from build123d import *

# Parameters (mm, degrees)
BOSS_EXTRUDE1_DEPTH        = 6.35
SKETCH2_R                  = 7
MOTOR_BEARING_HOLES_DEPTH  = 135.10382172
SKETCH3_R                  = 14.2875
CUT_EXTRUDE1_DEPTH         = 135.10382172
SKETCH4_R                  = 14.2875
CUT_EXTRUDE2_DEPTH         = 135.10382172
SKETCH5_R                  = 4.7625
CUT_EXTRUDE3_DEPTH         = 50.8
F_10_CLEARANCE_HOLE1_D     = 5.1054
F_10_CLEARANCE_HOLE2_D     = 5.1054
F_10_CLEARANCE_HOLE2_DEPTH = 50.8
F_10_CLEARANCE_HOLE2_TIP   = 1.533816902
FILLET1_R                  = 6.35
SKETCH10_R                 = 4.7625
CUT_EXTRUDE4_DEPTH         = 50.8


with BuildPart() as part:
    # Sketch1 → Boss-Extrude1 (new body)
    with BuildSketch(Plane(origin=(0, 0, 0), x_dir=(1, 0, 0), z_dir=(0, 1, 0))):
        Polygon((-69.85, -19.05), (69.85, -19.05), (69.85, 57.15), (6.35, 114.3), (-6.35, 114.3), (-69.85, 57.15), align=None)
    extrude(amount=BOSS_EXTRUDE1_DEPTH)

    # Sketch2 → Motor Bearing Holes (cut, through all)
    with BuildSketch(Plane(origin=(0, 6.35, 0), x_dir=(1, 0, 0), z_dir=(0, 1, 0))):
        with Locations(Location((-34.29, 25.4, 0), (0, 0, 270))):
            Circle(SKETCH2_R)
        with Locations(Location((34.29, 25.4, 0), (0, 0, 270))):
            Circle(SKETCH2_R)
    extrude(amount=-MOTOR_BEARING_HOLES_DEPTH, mode=Mode.SUBTRACT)

    # Sketch3 → Cut-Extrude1 (cut, through all)
    with BuildSketch(Plane(origin=(0, 6.35, 0), x_dir=(1, 0, 0), z_dir=(0, 1, 0))):
        with Locations(Location((0, 25.4, 0), (0, 0, 270))):
            Circle(SKETCH3_R)
    extrude(amount=-CUT_EXTRUDE1_DEPTH, mode=Mode.SUBTRACT)

    # Sketch4 → Cut-Extrude2 (cut, through all)
    with BuildSketch(Plane(origin=(0, 6.35, 0), x_dir=(1, 0, 0), z_dir=(0, 1, 0))):
        with Locations(Location((0, 63.5, 0), (0, 0, 270))):
            Circle(SKETCH4_R)
    extrude(amount=-CUT_EXTRUDE2_DEPTH, mode=Mode.SUBTRACT)

    # Sketch5 → Cut-Extrude3 (cut)
    with BuildSketch(Plane(origin=(0, 38.1, 19.05), x_dir=(-0.9584281674521108, 0, 0.2853339233851958), z_dir=(0, 1, 0))):
        with Locations(Location((21.697168114, -77.740965053, 0), (0, 0, 73.42119018))):
            Circle(SKETCH5_R)
        with Locations(Location((18.665649821, -27.031499499, 0), (0, 0, 73.42119018))):
            Circle(SKETCH5_R)
        with Locations(Location((-30.411025551, -12.420868461, 0), (0, 0, 73.42119018))):
            Circle(SKETCH5_R)
        with Locations(Location((-60.684163962, -53.21519516, 0), (0, 0, 73.42119018))):
            Circle(SKETCH5_R)
    extrude(amount=-CUT_EXTRUDE3_DEPTH, mode=Mode.SUBTRACT)

    # #10 Clearance Hole1 (through all)
    with Locations(Plane(origin=(0, 6.35, 19.05), x_dir=(1, 0, 0), z_dir=(0, 1, 0))):
        with Locations((-63.5, 6.35), (63.5, 6.35), (0, 107.95)):
            Hole(F_10_CLEARANCE_HOLE1_D / 2)

    # #10 Clearance Hole2
    with Locations(Plane(origin=(0, 38.1, 19.05), x_dir=(1, 0, 0), z_dir=(0, 1, 0))):
        with Locations((-63.5, 31.75), (63.5, 31.75), (0, 127)):
            Hole(F_10_CLEARANCE_HOLE2_D / 2, depth=F_10_CLEARANCE_HOLE2_DEPTH)
            with Locations((0, 0, -(F_10_CLEARANCE_HOLE2_DEPTH + F_10_CLEARANCE_HOLE2_TIP / 2))):  # 118° drill point
                Cone(0, F_10_CLEARANCE_HOLE2_D / 2, F_10_CLEARANCE_HOLE2_TIP, mode=Mode.SUBTRACT)

    # Fillet1
    fillet1_edges = [part.edges().sort_by_distance(p)[0] for p in [
        (-69.85, 3.175, -57.15),
        (-6.35, 3.175, -114.3),
        (6.35, 3.175, -114.3),
        (69.85, 3.175, -57.15),
        (69.85, 3.175, 19.05),
        (-69.85, 3.175, 19.05),
    ]]
    fillet(fillet1_edges, radius=FILLET1_R)

    # Sketch10 → Cut-Extrude4 (cut)
    with BuildSketch(Plane(origin=(0, -28.575, 19.05), x_dir=(-1, 0, 0), z_dir=(0, -1, 0))):
        with Locations(Location((-44.45, 85.725, 0), (0, 0, 270))):
            Circle(SKETCH10_R)
        with Locations(Location((44.45, 85.725, 0), (0, 0, 270))):
            Circle(SKETCH10_R)
        with Locations(Location((0, 6.35, 0), (0, 0, 270))):
            Circle(SKETCH10_R)
    extrude(amount=-CUT_EXTRUDE4_DEPTH, mode=Mode.SUBTRACT)


solid = part.part
Design review of the part built by this model. Coordinates are the model's own, in mm. Coordinates: 2 decimals unless noted, no trailing zeros. Order: outer loops, then holes, each group sorted by start corner. A loop starts at its lowest first (then second) coordinate and runs counter-clockwise, first axis right, second up. Notation, with made-up numbers: (6, 18.25) -> (48, 18.25) arc R27 ccw to (48, 50.25) -> close; hole circle Ø8 at (-6, -13). An arc over 180 degrees is marked (long way). Use one line per item in the form item = value. Start each with the question number.
(1) Add section D-D on y = 1.25. Give the number of separate pieces and of enclosed holes in the cut face, plus the area to 3 significant figures.
(2) For probe 1 along X at (y, z) = (3, -25.4); probe 2 along X at (y, z) = (5.25, -22); probe 3 along Z at (x, y) = (-42, 5.75) (3 decimals), list the stretches that pass through material, from the lowest coordinate up.
(3) Insertion check: pin 1 (15 mm diameter, centred on x = -42.98, z = -49.27, fed in from +Y). The pin has a flat end and moves straight along its axis. Give the tip position at first contact, or say it passes through.
(4) Add section C-C on z = -23. State the section outline as (x, y) points, plus the area to 3 significant figures.
(5) Add section B-B on x = -34.29. State the section outline as (y, z) points, plus the area to 3 significant figures.
(6) Add section A-A on z = -107.95. State the section outline as (x, y) points.
(7) The part is to be moulded in two halves that separate along X. For faces 1 (the cylindrical face through (-40.5, 3.22, -22.17)), 2 (the flat face through (15, 6.35, -34)), 3 (the flat face through (-37.54, 3.13, -86.23)), say which applies: +X half, -X half, draft (parallel to the pull), parting line (faces both ways), or undercut.
Answer block:
q1.separate_pieces = 1
q1.enclosed_holes = 17
q1.area = 12,800 mm²
q2.probe_1 = -69.85 to -41.29, -27.29 to -14.29, 14.29 to 27.29, 41.29 to 69.85
q2.probe_2 = -69.85 to -40.41, -28.17 to -13.88, 13.88 to 28.17, 40.41 to 69.85
q2.probe_3 = -82.215 to -70.759, -62.591 to -53.929, -44.607 to 19.05
q3.pin_1 = 6.35
q4.outline = (-69.85, 0) -> (-40.87, 0) -> (-40.87, 6.35) -> (-69.85, 6.35) -> close; (-27.71, 0) -> (-14.08, 0) -> (-14.08, 6.35) -> (-27.71, 6.35) -> close; (14.08, 0) -> (27.71, 0) -> (27.71, 6.35) -> (14.08, 6.35) -> close; (40.87, 0) -> (69.85, 0) -> (69.85, 6.35) -> (40.87, 6.35) -> close
q4.area = 541 mm²
q5.outline = (0, -89.15) -> (6.35, -89.15) -> (6.35, -32.4) -> (0, -32.4) -> close; (0, -18.4) -> (6.35, -18.4) -> (6.35, 19.05) -> (0, 19.05) -> close
q5.area = 598 mm²
q6.outline = (-13.41, 0) -> (-2.55, 0) -> (-2.55, 6.35) -> (-13.41, 6.35) -> close; (2.55, 0) -> (13.41, 0) -> (13.41, 6.35) -> (2.55, 6.35) -> close
q7.face_1 = undercut
q7.face_2 = draft
q7.face_3 = -X half
